from build123d import *

# Parameters (mm, degrees)
F0_W     = 20
F0_H     = 80
F1_DEPTH = 25
F2_R     = 4
F3_DEPTH = 25
F4_R     = 5


with BuildPart() as f1:
    # F0 (on Front) → F1 (new body)
    with BuildSketch(Plane.XZ):
        Rectangle(F0_W, F0_H)
    extrude(amount=F1_DEPTH)

    # F2 (on face) → F3 (cut)
    with BuildSketch(Plane.XZ.offset(25)):
        with Locations((0, 30)):
            Circle(F2_R)
    extrude(amount=-F3_DEPTH, mode=Mode.SUBTRACT)

    # F4
    f4_edges = [f1.edges().sort_by_distance(p)[0] for p in [
        (0, -25, 40),
        (10, -12.5, 40),
        (0, 0, 40),
        (-10, -12.5, 40),
        (10, -25, 0),
        (-10, 0, 0),
        (10, 0, 0),
        (-10, -25, 0),
    ]]
    fillet(f4_edges, radius=F4_R)


solid = f1.part
For this review, take the finished solid that the model builds, in its own axes (mm). Round coordinates to 2 decimals unless told otherwise and drop trailing zeros. Loops run counter-clockwise (first coordinate to the right, second up) from the corner with the lowest first, then second, coordinate; pieces in that order, holes last. Notation, with made-up numbers: (34.25, 60.25) - (38.25, 60.25) arc R13 ccw to (38.25, 75.25) - close; hole circle Ø2 at (-34, 28.5). An arc over 180 degrees is marked (long way). Use one line per item in the form item = value.
1) We need section A-A on z = 30. Write out the cut boundary in (x, y).
Solutions:
outline = (-10, -20) arc R5 ccw to (-5, -25) - (-4, -25) - (-4, 0) - (-5, 0) arc R5 ccw to (-10, -5) - close; (4, -25) - (5, -25) arc R5 ccw to (10, -20) - (10, -5) arc R5 ccw to (5, 0) - (4, 0) - close
2) We need section D-D on x = -8. Write out the cut boundary in (y, z), then the cut area to 3 significant figures.
Solutions:
outline = (-24, -40) - (-1, -40) - (-1, 35) arc R4 ccw to (-5, 39) - (-20, 39) arc R4 ccw to (-24, 35) - close
area = 1,810 mm2
3) Mouldability with a two-part tool opening along X and no side actions: class faces 1 (the face through (0, -12, -40)), 2 (the face through (10, -12, -3)), 3 (the face through (-0.521, -12.675, 33.966)) as pulls with the +X half, pulls with the -X half, needs draft (parallel to the pull), parting line crosses it, or undercut.
Solutions:
face_1 = needs draft
face_2 = pulls with the +X half
face_3 = undercut
4) We need section C-C on x = 0. Write out the cut boundary in (y, z).
Solutions:
outline = (-25, -40) - (0, -40) - (0, 26) - (-25, 26) - close; (-25, 34) - (0, 34) - (0, 35) arc R5 ccw to (-5, 40) - (-20, 40) arc R5 ccw to (-25, 35) - close
5) We need section B-B on y = -17.5. Write out the cut boundary in (x, z), then the cut area to 3 significant figures.
Solutions:
outline = (-10, -40) - (10, -40) - (10, 35) arc R5 ccw to (5, 40) - (-5, 40) arc R5 ccw to (-10, 35) - close; hole circle Ø8 at (0, 30)
area = 1,540 mm2
6) Wall thickness on probe 1 along Z at (x, y) = (0, -12.75); probe 2 along Z at (x, y) = (1.75, -22.5); probe 3 along Y at (x, z) = (7.25, -13): over which ranges is each line inside the solid? List them lowest first.
Solutions:
probe_1 = -40 to 26, 34 to 40
probe_2 = -40 to 26.4, 33.6 to 39.33
probe_3 = -24.47 to -0.53
7) Clearance check with flat-ended pins moving along their axes: P1, Ø1.5, axis at x = 7.5, z = -19, coming from the +Y side; P2, Ø1.5, axis at x = 6.5, z = -0.5, coming from the +Y side. State where each tip first meets the part, or that it passes through.
Solutions:
P1 = -0.32
P2 = -0.06
